Verification items for the finished model (mm, model axes). A direction names the side the tool comes from. Round coordinates to 2 decimals unless told otherwise and drop trailing zeros. Write item = value, one per line. Start each with the question number.
from build123d import *

# Parameters (mm, degrees)
SKETCH1_W           = 598
SKETCH1_H           = 192
BOSS_EXTRUDE1_DEPTH = 18
SKETCH2_W           = 87.4
SKETCH2_H           = 87.6
SKETCH2_W_2         = 79.646425984
SKETCH2_H_2         = 79.646425984
CUT_EXTRUDE1_DEPTH  = 7
CUT_EXTRUDE2_DEPTH  = 10.5


with BuildPart() as part:
    # Sketch1 → Boss-Extrude1 (new body)
    with BuildSketch(Plane.XY):
        Rectangle(SKETCH1_W, SKETCH1_H)
    extrude(amount=BOSS_EXTRUDE1_DEPTH)

    # Sketch2 → Cut-Extrude1 (cut)
    with BuildSketch(Plane.XY.offset(18)):
        Rectangle(SKETCH2_W, SKETCH2_H)
        Rectangle(SKETCH2_W_2, SKETCH2_H_2, mode=Mode.SUBTRACT)
    extrude(amount=-CUT_EXTRUDE1_DEPTH, mode=Mode.SUBTRACT)

    # Sketch3 → Cut-Extrude2 (cut)
    with BuildSketch(Plane.XY.offset(11)):
        with BuildLine():
            Line((30, -33.2), (-30, -33.2))
            Line((-30, -33.2), (-30, -5.0989999))
            ThreePointArc((-30, -5.0989999), (-25.197000899, -0.1), (-30, 4.8989999))
            Line((-30, 4.8989999), (-30, 33.8))
            Line((-30, 33.8), (30, 33.8))
            Line((30, 33.8), (30, 4.8989999))
            ThreePointArc((30, 4.8989999), (25.197000899, -0.1), (30, -5.0989999))
            Line((30, -5.0989999), (30, -33.2))
        make_face()
        with BuildLine():
            Line((26.16375103, -28.91618865), (-26.16375103, -28.91618865))
            Line((-26.16375103, -28.91618865), (-26.16375103, -8.093369002))
            ThreePointArc((-26.16375103, -8.093369002), (-21.245378078, -0.1), (-26.16375103, 7.893369002))
            Line((-26.16375103, 7.893369002), (-26.16375103, 29.51618865))
            Line((-26.16375103, 29.51618865), (26.16375103, 29.51618865))
            Line((26.16375103, 29.51618865), (26.16375103, 7.893369002))
            ThreePointArc((26.16375103, 7.893369002), (21.245378078, -0.1), (26.16375103, -8.093369002))
            Line((26.16375103, -8.093369002), (26.16375103, -28.91618865))
        make_face(mode=Mode.SUBTRACT)
    extrude(amount=-CUT_EXTRUDE2_DEPTH, mode=Mode.SUBTRACT)


solid = part.part
1) Access from +Z, -Z, +X, -X, +Y, -Y to the whole of each face (thin tool, end or side, straight path). Record for faces 1 (the flat face through (-1, 1, 18)), 2 (the flat face through (-26.164, 19, 6)).
2) Gauge pin test, flat end, axial feed: P1, Ø12, axis at x = -43, y = -38, coming from the +Z side. Record the tip position at first contact, or that the pin passes through.
3) Release check for a two-part mould opening along X. For faces 3 (the flat face through (-3, -42, 11)), 4 (the flat face through (-299, -1, 9)), 5 (the flat face through (-4, 44, 18)) record: pulls with the +X half, pulls with the -X half, needs draft (parallel to the pull), parting line crosses it, or undercut.
4) Scan lines: probe 1 along X at (y, z) = (-16, 3); probe 2 along X at (y, z) = (9, 16.75); probe 3 along X at (y, z) = (-40, 14.5). Record each from-to range of solid material in increasing order.
Geometry results:
q1.face_1 = +Z, +X, -X, +Y, -Y
q1.face_2 = none
q2.P1 = 18
q3.face_3 = undercut
q3.face_4 = pulls with the -X half
q3.face_5 = needs draft
q4.probe_1 = -299 to -30, -26.16 to 26.16, 30 to 299
q4.probe_2 = -299 to -43.7, -39.82 to 39.82, 43.7 to 299
q4.probe_3 = -299 to -43.7, 43.7 to 299
